Geometry: final body of the model. Coordinates: model frame, mm. A direction names the side the tool comes from. Round coordinates to 2 decimals unless told otherwise and drop trailing zeros. Loops run counter-clockwise (first coordinate to the right, second up) from the corner with the lowest first, then second, coordinate; pieces in that order, holes last. Notation, with made-up numbers: (5, -17.75) - (27, -17.75) arc R27 ccw to (27, 20.25) - close; hole circle Ø3 at (-13.75, 29.25). An arc over 180 degrees is marked (long way). Write item = value, one per line. Start each with the question number.
Item 1: Section D-D (x = 13.5). Return loops of the section in (y, z), plus the area to 3 significant figures.
Item 2: Draft query along Z for faces 3 (the flat face through (4, -12.7, 2)), 4 (the flat face through (17, -7, 77.498)), 5 (the flat face through (56, -4, 13.998)). Return one class per face: pulls with the +Z half, pulls with the -Z half, needs draft (parallel to the pull), parting line crosses it, or undercut.
Item 3: Access query for faces 1 (the cylindrical face through (52.585, -12.281, -62.024)), 2 (the flat face through (56, -4, -49.502)). Directions: +Z, -Z, +X, -X, +Y, -Y. A direction counts if a zero-diameter tool reaches every point of the face in a straight line with its end or side. Return the directions, or none.
Item 4: Section B-B (x = 57.5). Return loops of the section in (y, z).
Item 5: Line query: line 1 (Z direction, x = 58, y = -2.75); line 2 (Y direction, x = -2.5, z = 26.5); line 3 (X direction, y = -17, z = 59). Output: solid intervals per line, ascending. Write a range as from..to.
Item 6: First-contact query: pin 1 (1 mm diameter, centred on x = 32, z = -8, fed in from -Y); pin 2 (4 mm diameter, centred on y = -5, z = -26, fed in from +X). Flat tips, straight axial feed; report the tip coordinate or a pass-through.
Item 7: Section A-A (z = 11.5). Return loops of the section in (x, y) (3 decimals).
Item 8: Section C-C (y = -16.75). Return loops of the section in (x, z).
from build123d import *

# Parameters (mm, degrees)
F0_W     = 101.6
F0_H     = 152.4
F1_DEPTH = 12.7
F3_DEPTH = 152.4
F4_R     = 9.525
F5_DEPTH = 152.4
F7_W     = 50.8
F7_H     = 38.1
F8_DEPTH = 50.8


# Not quite as in the source:
# - a feature names something its author has since deleted; it is built from what else it names


with BuildPart() as f1:
    # F0 (on Front) → F1 (new body)
    with BuildSketch(Plane.XZ):
        with Locations((11.3006858155, 1.2977712616)):
            Rectangle(F0_W, F0_H)
    extrude(amount=F1_DEPTH)

    # F2 (on face) → F3 (join)
    with BuildSketch(Plane.XY.offset(77.4977712616)):
        with BuildLine():
            ThreePointArc((49.4006858155, -12.7), (62.1006858155, -25.4), (74.8006858155, -12.7))
            ThreePointArc((74.8006858155, -12.7), (71.0809419366, -3.7197438789), (62.1006858155, 0))
            Line((62.1006858155, 0), (62.1006858155, -12.7))
            Line((62.1006858155, -12.7), (49.4006858155, -12.7))
        make_face()
    extrude(amount=-F3_DEPTH)

    # F4 (on face) → F5 (cut, through all)
    with BuildSketch(Plane.XY.offset(77.4977712616)):
        with Locations((62.1006858155, -12.7)):
            Circle(F4_R)
    extrude(amount=-F5_DEPTH, mode=Mode.SUBTRACT)

    # F7 (on offset) → F8 (cut)
    with BuildSketch(Plane.XZ.offset(25.4)):
        with Locations((74.8006858155, 33.0477712616)):
            Rectangle(F7_W, F7_H)
        with Locations((74.8006858155, -30.4522287384)):
            Rectangle(F7_W, F7_H)
    extrude(amount=-F8_DEPTH, mode=Mode.SUBTRACT)


solid = f1.part
Taken from the geometry:
q1.outline = (-12.7, -74.9) - (0, -74.9) - (0, 77.5) - (-12.7, 77.5) - close
q1.area = 1,940 mm^2
q2.face_3 = needs draft
q2.face_4 = pulls with the +Z half
q2.face_5 = undercut
q3.face_1 = +Z, -Z
q3.face_2 = +X, +Y, -Y
q4.outline = (-24.54, -74.9) - (-21.04, -74.9) - (-21.04, -49.5) - (-24.54, -49.5) - close; (-24.54, -11.4) - (-21.04, -11.4) - (-21.04, 14) - (-24.54, 14) - close; (-24.54, 52.1) - (-21.04, 52.1) - (-21.04, 77.5) - (-24.54, 77.5) - close; (-4.36, -74.9) - (0, -74.9) - (0, -49.5) - (-4.36, -49.5) - close; (-4.36, -11.4) - (0, -11.4) - (0, 14) - (-4.36, 14) - close; (-4.36, 52.1) - (0, 52.1) - (0, 77.5) - (-4.36, 77.5) - close
q5.line_1 = -74.9..-49.5, -11.4..14, 52.1..77.5
q5.line_2 = -12.7..0
q5.line_3 = 50.15..53.6, 70.6..74.05
q6.pin_1 = -12.7
q6.pin_2 = 49.4
q7.outline = (-39.499, -12.7) - (49.401, -12.7) arc R12.7 ccw (long way) to (62.101, 0) - (-39.499, 0) - close; hole circle Ø19.05 at (62.101, -12.7)
q8.outline = (50.06, -74.9) - (53.48, -74.9) - (53.48, -49.5) - (50.06, -49.5) - close; (50.06, -11.4) - (53.48, -11.4) - (53.48, 14) - (50.06, 14) - close; (50.06, 52.1) - (53.48, 52.1) - (53.48, 77.5) - (50.06, 77.5) - close; (70.72, -74.9) - (74.14, -74.9) - (74.14, -49.5) - (70.72, -49.5) - close; (70.72, -11.4) - (74.14, -11.4) - (74.14, 14) - (70.72, 14) - close; (70.72, 52.1) - (74.14, 52.1) - (74.14, 77.5) - (70.72, 77.5) - close
